```python
from build123d import *
from OCP.BRepFilletAPI import BRepFilletAPI_MakeChamfer

# Parameters (mm, degrees)
SKETCH_1_W          = 170
SKETCH_1_H          = 80
SKETCH_1_R          = 2
EXTRUDE_1_DEPTH     = 3
SKETCH_2_R          = 1.5
SKETCH_2_W          = 90
SKETCH_2_H          = 60
CUT_EXTRUDE_1_DEPTH = 188.906891837
SKETCH_3_R          = 1.5
CUT_EXTRUDE_2_DEPTH = 5
CUT_EXTRUDE_3_DEPTH = 10
CHAMFER_1_SIZE      = 2
CHAMFER_1_SIZE2     = 3.464101615
CHAMFER_2_SIZE      = 8
CHAMFER_2_SIZE2     = 13.856406461


with BuildPart() as part:
    # 草图1 → 凸台-拉伸1 (new body)
    with BuildSketch(Plane(origin=(0, 0, 0), x_dir=(1, 0, 0), z_dir=(0, 1, 0))):
        with Locations((85, 40)):
            Rectangle(SKETCH_1_W, SKETCH_1_H)
        with Locations(Location((10, 65, 0), (0, 0, 270))):
            Circle(SKETCH_1_R, mode=Mode.SUBTRACT)
        with Locations(Location((10, 15, 0), (0, 0, 90))):
            Circle(SKETCH_1_R, mode=Mode.SUBTRACT)
        with Locations(Location((160, 15, 0), (0, 0, 270))):
            Circle(SKETCH_1_R, mode=Mode.SUBTRACT)
        with Locations(Location((160, 65, 0), (0, 0, 90))):
            Circle(SKETCH_1_R, mode=Mode.SUBTRACT)
    extrude(amount=EXTRUDE_1_DEPTH)

    # 草图2 → 切除-拉伸1 (cut, through all)
    with BuildSketch(Plane(origin=(0, 3, 0), x_dir=(1, 0, 0), z_dir=(0, 1, 0))):
        with Locations(Location((35, 45, 0), (0, 0, 270))):
            Circle(SKETCH_2_R)
        with Locations(Location((35, 5, 0), (0, 0, 270))):
            Circle(SKETCH_2_R)
        with Locations(Location((135, 5, 0), (0, 0, 90))):
            Circle(SKETCH_2_R)
        with Locations(Location((135, 45, 0), (0, 0, 90))):
            Circle(SKETCH_2_R)
        with Locations(Location((45, 63, 0), (0, 0, 270))):
            Circle(SKETCH_2_R)
        with Locations(Location((65, 63, 0), (0, 0, 270))):
            Circle(SKETCH_2_R)
        with Locations(Location((105, 63, 0), (0, 0, 90))):
            Circle(SKETCH_2_R)
        with Locations(Location((125, 63, 0), (0, 0, 90))):
            Circle(SKETCH_2_R)
        with Locations((85, 30)):
            Rectangle(SKETCH_2_W, SKETCH_2_H)
    extrude(amount=-CUT_EXTRUDE_1_DEPTH, mode=Mode.SUBTRACT)

    # 草图3 → 切除-拉伸2 (cut)
    with BuildSketch(Plane(origin=(0, 3, 0), x_dir=(1, 0, 0), z_dir=(0, 1, 0))):
        with Locations(Location((32, 15, 0), (0, 0, 270))):
            Circle(SKETCH_3_R)
        with Locations(Location((32, 35, 0), (0, 0, 270))):
            Circle(SKETCH_3_R)
    extrude(amount=-CUT_EXTRUDE_2_DEPTH, mode=Mode.SUBTRACT)

    # 草图5 → 切除-拉伸3 (cut)
    with BuildSketch(Plane(origin=(0, 3, 0), x_dir=(1, 0, 0), z_dir=(0, 1, 0))):
        Polygon((15.391630359, 28.000778829), (25.783260719, 34.000389415), (25.783260719, 45.999610585), (15.391630359, 51.999221171), (5, 45.999610585), (5, 34.000389415), align=None)
        Polygon((35, 60), (35, 70), (26.339745962, 75), (17.679491924, 70), (17.679491924, 60), (26.339745962, 55), align=None)
        Polygon((21, 13), (25.330127019, 15.5), (25.330127019, 20.5), (21, 23), (16.669872981, 20.5), (16.669872981, 15.5), align=None)
        Polygon((153.330127019, 15.5), (149, 13), (144.669872981, 15.5), (144.669872981, 20.5), (149, 23), (153.330127019, 20.5), align=None)
        Polygon((143.660254038, 55), (135, 60), (135, 70), (143.660254038, 75), (152.320508076, 70), (152.320508076, 60), align=None)
        Polygon((165, 34.000389415), (154.608369641, 28.000778829), (144.216739281, 34.000389415), (144.216739281, 45.999610585), (154.608369641, 51.999221171), (165, 45.999610585), align=None)
    extrude(amount=-CUT_EXTRUDE_3_DEPTH, mode=Mode.SUBTRACT)

    # 倒角1: one chamfer whose edges measure the first distance from different faces: ONE call of the kernel's chamfer builder (chamfer() names one face for all edges)
    chamfer_1_edges_1 = [part.edges().sort_by_distance(p)[0] for p in [
        (40, 1.5, 0),
        (40, 1.5, -60),
    ]]
    chamfer_1_side_1 = [part.faces().sort_by_distance(p)[0] for p in [
        (40, 1.5, -30),
    ]]
    chamfer_1_edges_2 = [part.edges().sort_by_distance(p)[0] for p in [
        (130, 1.5, -60),
        (130, 1.5, 0),
    ]]
    chamfer_1_side_2 = [part.faces().sort_by_distance(p)[0] for p in [
        (130, 1.5, -30),
    ]]
    chamfer_1 = BRepFilletAPI_MakeChamfer(part.part.solid().wrapped)
    for e in chamfer_1_edges_1:
        chamfer_1.Add(CHAMFER_1_SIZE, CHAMFER_1_SIZE2, e.wrapped, chamfer_1_side_1[0].wrapped)  # the first distance lies on this face
    for e in chamfer_1_edges_2:
        chamfer_1.Add(CHAMFER_1_SIZE, CHAMFER_1_SIZE2, e.wrapped, chamfer_1_side_2[0].wrapped)  # the first distance lies on this face
    add(Compound.cast(chamfer_1.Shape()), mode=Mode.REPLACE)

    # 倒角2: one chamfer whose edges measure the first distance from different faces: ONE call of the kernel's chamfer builder (chamfer() names one face for all edges)
    chamfer_2_edges_1 = [part.edges().sort_by_distance(p)[0] for p in [
        (0, 1.5, -80),
        (0, 1.5, 0),
    ]]
    chamfer_2_side_1 = [part.faces().sort_by_distance(p)[0] for p in [
        (0, 1.5, -40),
    ]]
    chamfer_2_edges_2 = [part.edges().sort_by_distance(p)[0] for p in [
        (170, 1.5, -80),
        (170, 1.5, 0),
    ]]
    chamfer_2_side_2 = [part.faces().sort_by_distance(p)[0] for p in [
        (170, 1.5, -40),
    ]]
    chamfer_2 = BRepFilletAPI_MakeChamfer(part.part.solid().wrapped)
    for e in chamfer_2_edges_1:
        chamfer_2.Add(CHAMFER_2_SIZE, CHAMFER_2_SIZE2, e.wrapped, chamfer_2_side_1[0].wrapped)  # the first distance lies on this face
    for e in chamfer_2_edges_2:
        chamfer_2.Add(CHAMFER_2_SIZE, CHAMFER_2_SIZE2, e.wrapped, chamfer_2_side_2[0].wrapped)  # the first distance lies on this face
    add(Compound.cast(chamfer_2.Shape()), mode=Mode.REPLACE)


solid = part.part
```
The listing builds one solid part. Answer for the finished solid, in the listing's coordinates (mm). A direction names the side the tool comes from. Give positions to 0.01 mm unless a question says otherwise; leave off trailing zeros. Order: outer loops, then holes, each group sorted by start corner. A loop starts at its lowest first (then second) coordinate and runs counter-clockwise, first axis right, second up. Notation, with made-up numbers: M 65.5,26 L 89.5,26 A36 cw 89.5,63 Z; hole C -12.5,48.5 d7. An arc over 180 degrees is marked long. Put each result on its own line as item: value. Start each with the question number.
Item 1: The part is cut by section B-B, the plane y = 0.5. State how many separate pieces and enclosed holes the cut face has, and give its area (3 significant figures).
Item 2: Find the intervals of material crossed by line 1 along X through (y, z) = (2.65, -43); line 2 along X through (y, z) = (1, -65); line 3 along X through (y, z) = (2.25, -35), in increasing order.
Item 3: The part is cut by section A-A, the plane x = 160. Determine the outline of the cut face in (y, z).
Item 4: The part is cut by section C-C, the plane x = 69. Determine the outline of the cut face in (y, z), and give its area (3 significant figures).
Item 5: For a pull along Z with two mould halves and no side action, classify faces 4 (the face through (123.735, 1.521, -63.806)), 5 (the face through (84, 0, -67)), 6 (the face through (84, 1, -80)) as +Z half, -Z half, draft (parallel to the pull), parting line (faces both ways), or undercut.
Item 6: Which of the six approach directions +Z, -Z, +X, -X, +Y, -Y give full straight-line access (tool end or side, diameter ignored) to faces 1 (the face through (130, 2, -30)), 2 (the face through (0, 1, -40)), 3 (the face through (144.67, 2, -18))?
Item 7: A flat-ended cylindrical pin translates along its axis: P1, Ø3, axis at x = 160, z = -65, coming from the +Y side. Find the tip coordinate at first contact, or state that the pin passes through.
Answer key:
1. separate pieces: 1
1. enclosed holes: 20
1. area: 6,460 mm²
2. line 1: x = 0 to 5, 25.78 to 40, 130 to 144.22, 165 to 170
2. line 2: x = 0 to 8, 12 to 17.68, 35 to 135, 152.32 to 158, 162 to 170
2. line 3: x = 0 to 5, 25.78 to 30.5, 33.5 to 40, 130 to 144.22, 165 to 170
3. outline: M 0,-77.77 L 3,-77.77 L 3,-67 L 0,-67 Z; M 0,-63 L 3,-63 L 3,-48.89 L 0,-48.89 Z; M 0,-31.11 L 3,-31.11 L 3,-17 L 0,-17 Z; M 0,-13 L 3,-13 L 3,-2.23 L 0,-2.23 Z
4. outline: M 0,-80 L 3,-80 L 3,-60 L 0,-60 Z
4. area: 60.0 mm²
5. face 4: undercut
5. face 5: draft
5. face 6: -Z half
6. face 1: +Z, +Y, -Y
6. face 2: +Z, -Z, -X, +Y, -Y
6. face 3: +Y, -Y
7. P1: passes through
